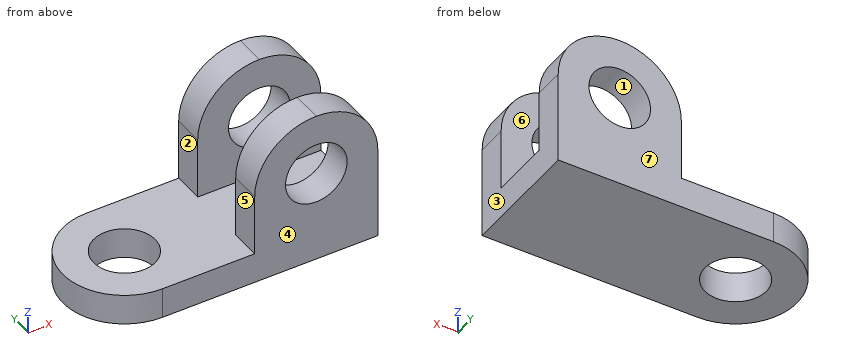
from build123d import *

# Parameters (mm, degrees)
F1_DEPTH = 12.7
F2_R     = 12.7
F3_DEPTH = 12.701
F4_W     = 50.8
F4_H     = 12.7
F5_DEPTH = 50.8
F6_R     = 12.7
F7_DEPTH = 50.801


with BuildPart() as f1:
    # F0 (on Top) → F1 (new body)
    with BuildSketch(Plane.XY):
        with BuildLine():
            ThreePointArc((25.4, 25.4), (17.960512, 7.439488), (0, 0))
            Line((0, 0), (88.9, 0))
            Line((88.9, 0), (88.9, 50.8))
            Line((88.9, 50.8), (0, 50.8))
            ThreePointArc((0, 50.8), (17.960512, 43.360512), (25.4, 25.4))
        make_face()
        with BuildLine():
            Line((0, 50.8), (0, 0))
            ThreePointArc((0, 0), (17.960512, 7.439488), (25.4, 25.4))
            ThreePointArc((25.4, 25.4), (17.960512, 43.360512), (0, 50.8))
        make_face()
        with BuildLine():
            ThreePointArc((0, 50.8), (-25.4, 25.4), (0, 0))
            Line((0, 0), (0, 50.8))
        make_face()
    extrude(amount=F1_DEPTH)

    # F2 (on face) → F3 (cut, through all)
    with BuildSketch(Plane.XY.offset(12.7)):
        with Locations((0, 25.4)):
            Circle(F2_R)
    extrude(amount=-F3_DEPTH, mode=Mode.SUBTRACT)

    # F4 (on face) → F5 (join)
    with BuildSketch(Plane.XY.offset(12.7)):
        with Locations((63.5, 44.45)):
            Rectangle(F4_W, F4_H)
        with Locations((63.5, 6.35)):
            Rectangle(F4_W, F4_H)
    extrude(amount=F5_DEPTH)

    # F6 (on face) → F7 (cut, through all)
    with BuildSketch(Plane.XZ):
        with BuildLine():
            ThreePointArc((63.5, 63.5), (81.460512, 56.060512), (88.9, 38.1))
            Line((88.9, 38.1), (88.9, 63.5))
            Line((88.9, 63.5), (63.5, 63.5))
        make_face()
        with BuildLine():
            ThreePointArc((38.1, 38.1), (45.539488, 56.060512), (63.5, 63.5))
            Line((63.5, 63.5), (38.1, 63.5))
            Line((38.1, 63.5), (38.1, 38.1))
        make_face()
        with Locations((63.5, 38.1)):
            Circle(F6_R)
    extrude(amount=-F7_DEPTH, mode=Mode.SUBTRACT)


solid = f1.part
Source: CAD feature listing. Evaluate the final solid. Frame: model axes, mm. Face numbers are marked on the shaded views. A direction names the side the tool comes from. Round coordinates to 2 decimals unless told otherwise and drop trailing zeros. Order: outer loops, then holes, each group sorted by start corner. A loop starts at its lowest first (then second) coordinate and runs counter-clockwise, first axis right, second up. Notation, with made-up numbers: (65, -12.5) - (107, -12.5) arc R35 ccw to (107, 25.5) - close; hole circle Ø3 at (40.25, 57.25). An arc over 180 degrees is marked (long way). Use a Markdown table: item, result. Add a question column.
1. Section query C-C (z = 35). Return the cut outline in (x, y).
2. Section query A-A (z = 14). Return the cut outline in (x, y).
3. Set-up query: the marked faces 5, 6 and 7. Return all of +Z, -Z, +X, -X, +Y, -Y with unobstructed straight access to the full face (end or side cutting, diameter ignored); none if empty.
4. Line query: probe 1 along Z at (x, y) = (63, 45); probe 2 along Y at (x, z) = (59, 56.5); probe 3 along Z at (x, y) = (12.5, 11.5). Output: solid intervals per line, ascending.
5. First-contact query: pin 1 (6.5 mm diameter, centred on y = 6.5, z = 28, fed in from -X); pin 2 (15 mm diameter, centred on x = 42, y = 29.5, fed in from +Z); pin 3 (4 mm diameter, centred on y = 12, z = 46, fed in from +X). Flat tips, straight axial feed; report the tip coordinate or a pass-through.
6. Mould query, pull axis X, two halves, no side actions, for the marked faces 1, 2, 3 and 4. Classes: +X half, -X half, draft (parallel to the pull), parting line (faces both ways), or undercut.
7. Section query B-B (x = 6). Return the cut outline in (y, z), then the cut area to 3 significant figures.
8. Section query D-D (y = 45.5). Return the cut outline in (x, z), then the cut area to 3 significant figures.
Derived:
| question | item | result |
|---|---|---|
| 1 | outline | (38.1, 0) - (51.18, 0) - (51.18, 12.7) - (38.1, 12.7) - close; (38.1, 38.1) - (51.18, 38.1) - (51.18, 50.8) - (38.1, 50.8) - close; (75.82, 0) - (88.9, 0) - (88.9, 12.7) - (75.82, 12.7) - close; (75.82, 38.1) - (88.9, 38.1) - (88.9, 50.8) - (75.82, 50.8) - close |
| 2 | outline | (38.1, 0) - (88.9, 0) - (88.9, 12.7) - (38.1, 12.7) - close; (38.1, 38.1) - (88.9, 38.1) - (88.9, 50.8) - (38.1, 50.8) - close |
| 3 | face 5 | +Z, -X, +Y, -Y |
| 3 | face 6 | +Z, +X, -X |
| 3 | face 7 | +Z, -Z, +X, -X, +Y |
| 4 | probe 1 | 0 to 25.41, 50.79 to 63.5 |
| 4 | probe 2 | 0 to 12.7, 38.1 to 50.8 |
| 4 | probe 3 | 0 to 12.7 |
| 5 | pin 1 | x = 38.1 |
| 5 | pin 2 | z = 12.7 |
| 5 | pin 3 | x = 88.21 |
| 6 | face 1 | undercut |
| 6 | face 2 | -X half |
| 6 | face 3 | +X half |
| 6 | face 4 | draft |
| 7 | outline | (0, 0) - (14.21, 0) - (14.21, 12.7) - (0, 12.7) - close; (36.59, 0) - (50.8, 0) - (50.8, 12.7) - (36.59, 12.7) - close |
| 7 | area | 361 mm2 |
| 8 | outline | (-15.53, 0) - (88.9, 0) - (88.9, 38.1) arc R25.4 ccw to (63.5, 63.5) arc R25.4 ccw to (38.1, 38.1) - (38.1, 12.7) - (-15.53, 12.7) - close; hole circle Ø25.4 at (63.5, 38.1) |
| 8 | area | 3,120 mm2 |
